Could you check a few things on this drawing? It's one solid part, dimensions in mm from its lowest x, y, z. A direction names the side the tool comes from. Give positions to 0.01 mm unless a question says otherwise; leave off trailing zeros. Loops run counter-clockwise (first coordinate to the right, second up) from the corner with the lowest first, then second, coordinate; pieces in that order, holes last. Notation, with made-up numbers: (2, 0) -> (6, 0) arc R7 cw to (6, 5) -> close; hole circle Ø1 at (-31, 4). An arc over 180 degrees is marked (long way). Use CSV: the item, a comma, the result in double quotes.
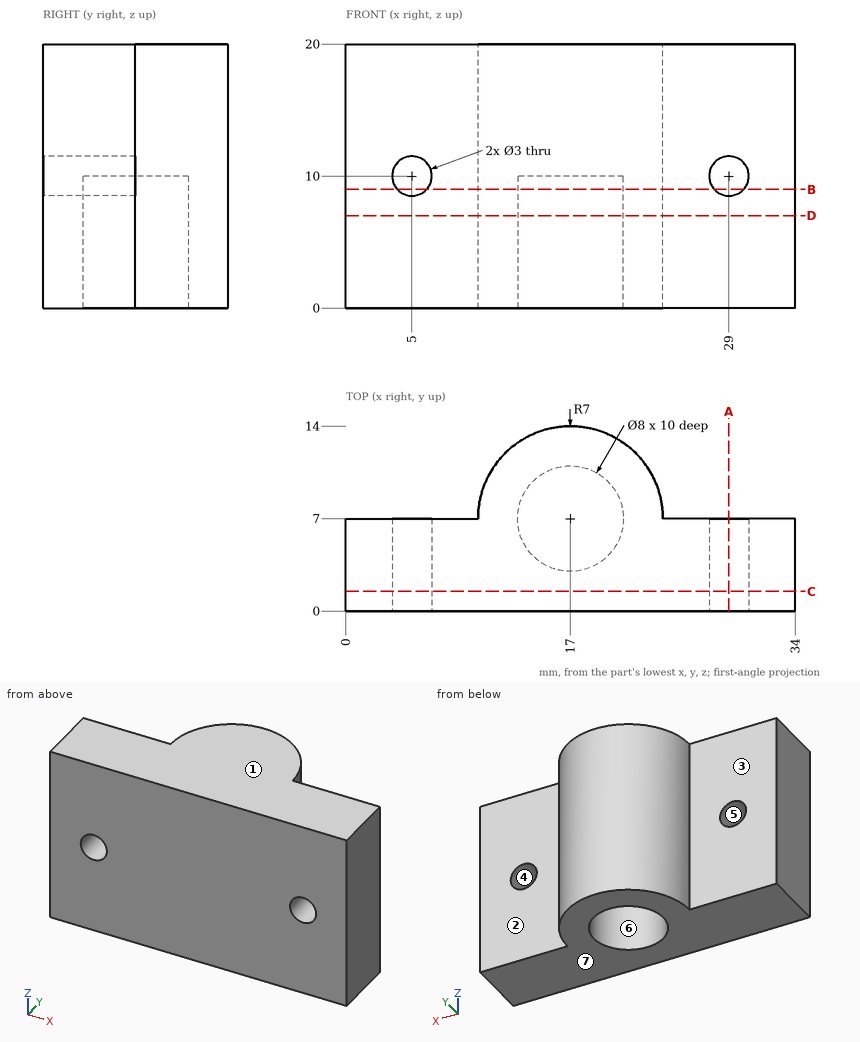
(1) If we section it at C-C, the plane y = 1.5: Write out the boundary of the cut face in (x, z), then the cut area to 3 significant figures.
Answer sheet:
outline,"(0, 0) -> (34, 0) -> (34, 20) -> (0, 20) -> close; hole circle Ø3 at (5, 10); hole circle Ø3 at (29, 10)"
area,"666 mm2"
(2) If I drill on L1, parallel to X at y = 1.75, z = 10; L2, parallel to Z at x = 29, y = 3; L3, parallel to Y at x = 17, z = 4.75, over which ranges is the centre line in solid material (lowest first)? Write a range as from..to.
Answer sheet:
L1,"x = 0..3.5, 6.5..27.5, 30.5..34"
L2,"z = 0..8.5, 11.5..20"
L3,"y = 0..3, 11..14"
(3) If we section it at B-B, the plane z = 9: Write out the boundary of the cut face in (x, y).
Answer sheet:
outline,"(0, 0) -> (3.88, 0) -> (3.88, 7) -> (0, 7) -> close; (6.12, 0) -> (27.88, 0) -> (27.88, 7) -> (24, 7) arc R7 ccw to (10, 7) -> (6.12, 7) -> close; (30.12, 0) -> (34, 0) -> (34, 7) -> (30.12, 7) -> close; hole circle Ø8 at (17, 7)"
(4) Will these pins go through, and if not, where does the flat tip stop? pin 1 Ø12 at (x, z) = (3.5, 2.5) entering from +Y; pin 2 Ø4 at (x, z) = (26.5, 9.5) entering from -Y; pin 3 Ø8 at (x, z) = (9, 11.5) entering from +Y; pin 4 Ø4 at (x, z) = (10.5, 8) entering from +Y.
Answer sheet:
pin 1,"stops at y = 7"
pin 2,"stops at y = 0"
pin 3,"stops at y = 12.74"
pin 4,"stops at y = 12.36"
(5) If we section it at A-A, the plane x = 29: Write out the boundary of the cut face in (y, z), then the cut area to 3 significant figures.
Answer sheet:
outline,"(0, 0) -> (7, 0) -> (7, 8.5) -> (0, 8.5) -> close; (0, 11.5) -> (7, 11.5) -> (7, 20) -> (0, 20) -> close"
area,"119 mm2"
(6) We'd pull the mould along Z, two halves only. Please class the marked faces 4, 5, 6 and 7: released by +Z, released by -Z, zero draft, split by the parting line, or undercut.
Answer sheet:
face 4,"undercut"
face 5,"undercut"
face 6,"zero draft"
face 7,"released by -Z"
(7) Which directions (+Z, -Z, +X, -X, +Y, -Y) give clear straight access to the entire face, cutting with the end or side of a thin tool? Please do the marked faces 1, 2 and 3.
Answer sheet:
face 1,"+Z, +X, -X, +Y, -Y"
face 2,"+Z, -Z, +X, +Y"
face 3,"+Z, -Z, -X, +Y"
(8) If we section it at D-D, the plane z = 7: Write out the boundary of the cut face in (x, y), then the cut area to 3 significant figures.
Answer sheet:
outline,"(0, 0) -> (34, 0) -> (34, 7) -> (24, 7) arc R7 ccw to (10, 7) -> (0, 7) -> close; hole circle Ø8 at (17, 7)"
area,"265 mm2"
